Here's the drawing with two shaded views (mm, measured from the low corner). I have some questions. Coordinates: 2 decimals unless noted, no trailing zeros. Write each loop counter-clockwise with the first axis right and the second up, starting at its lowest first coordinate (ties: lowest second). Pieces come first, ordered by that corner, then holes. Notation, with made-up numbers: (-28, -36.75) -> (1, -36.75) arc R21 cw to (1, -23.75) -> close; hole circle Ø1 at (65.5, 78). An arc over 180 degrees is marked (long way). Put each result on its own line as item: value. Start each with the question number.
Item 1: I want a section at D-D, the plane z = 126. List the corners of the cut face in (x, y) for me.
Item 2: I want a section at C-C, the plane z = 1155.5. List the corners of the cut face in (x, y) for me.
Item 3: I want a section at B-B, the plane x = 1826. List the corners of the cut face in (y, z) for me.
Item 4: If we mould it in two halves opening along X, with no side actions, what happens to the marked faces 1 and 2? For each: released by +X, released by -X, zero draft, split by the parting line, or undercut.
Item 5: I want a section at A-A, the plane y = 687. List the corners of the cut face in (x, z) for me.
Item 6: For pin 1 (2 mm diameter, centred on x = 584.5, y = 505.5, fed in from -Z), with a flat end and sliding along its axis, tell me the tip position at first contact or that it passes through.
Item 7: I need wall thicknesses on line 1 (X direction, y = 101.5, z = 893.5); line 2 (Z direction, x = 282, y = 480.5); line 3 (Y direction, x = 287, z = 61). Which ranges of each line are inside material? Lowest first, please. Write a range as [from, to].
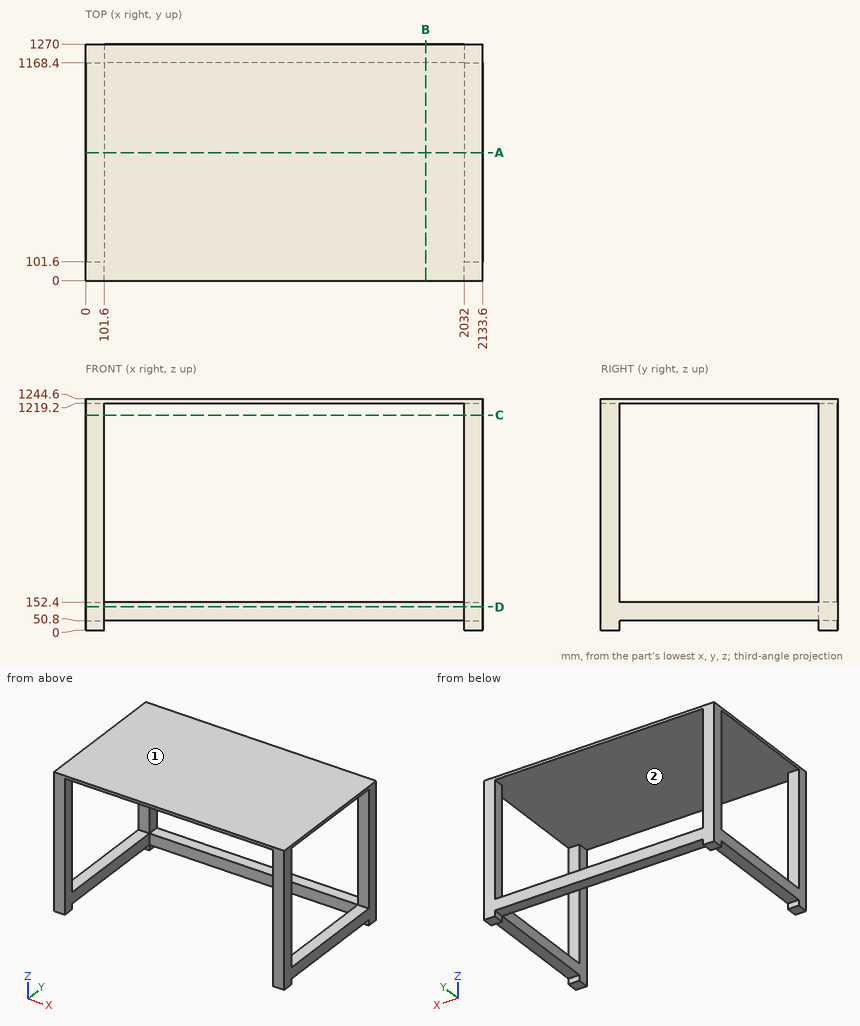
Calculated:
1. outline: (0, 0) -> (101.6, 0) -> (101.6, 1168.4) -> (2032, 1168.4) -> (2032, 0) -> (2133.6, 0) -> (2133.6, 1270) -> (0, 1270) -> close
2. outline: (0, 0) -> (101.6, 0) -> (101.6, 101.6) -> (0, 101.6) -> close; (0, 1168.4) -> (101.6, 1168.4) -> (101.6, 1270) -> (0, 1270) -> close; (2032, 0) -> (2133.6, 0) -> (2133.6, 101.6) -> (2032, 101.6) -> close; (2032, 1168.4) -> (2133.6, 1168.4) -> (2133.6, 1270) -> (2032, 1270) -> close
3. outline: (0, 1219.2) -> (1270, 1219.2) -> (1270, 1244.6) -> (0, 1244.6) -> close; (1168.4, 50.8) -> (1270, 50.8) -> (1270, 152.4) -> (1168.4, 152.4) -> close
4. face 1: zero draft
4. face 2: undercut
5. outline: (0, 50.8) -> (101.6, 50.8) -> (101.6, 152.4) -> (0, 152.4) -> close; (0, 1219.2) -> (2133.6, 1219.2) -> (2133.6, 1244.6) -> (0, 1244.6) -> close; (2032, 50.8) -> (2133.6, 50.8) -> (2133.6, 152.4) -> (2032, 152.4) -> close
6. pin 1: stops at z = 1219.2
7. line 1: x = [0, 101.6], [2032, 2133.6]
7. line 2: z = [1219.2, 1244.6]
7. line 3: y = [1168.4, 1270]
